from build123d import *

# Parameters (mm, degrees)
SKETCH1_R           = 10.16
BOSS_EXTRUDE4_DEPTH = 2.54
SKETCH1_7_R         = 10.16
BOSS_EXTRUDE5_DEPTH = 25.4
BOSS_EXTRUDE7_START = -27.94
SKETCH1_9_R         = 10.16
BOSS_EXTRUDE7_DEPTH = 2.54
FILLET1_R           = 0.508
FILLET2_R           = 0.508
FILLET3_R           = 0.508


with BuildPart() as part:
    # Sketch1 → Boss-Extrude4 (new body)
    # profile 1 of 4: a face of its own
    with BuildSketch(Plane(origin=(0, 0, 0), x_dir=(0, 0, -1), z_dir=(1, 0, 0))):
        with BuildLine():
            ThreePointArc((-12.743782522, 0.525454189), (-11.680659896, 5.122721879), (-9.018871744, 9.018871744))
            ThreePointArc((-9.018871744, 9.018871744), (-12.351999156, 6.704423948), (-16.283700751, 5.700367418))
            ThreePointArc((-16.283700751, 5.700367418), (-21.59, 0), (-16.283700751, -5.700367418))
            ThreePointArc((-16.283700751, -5.700367418), (-12.351999156, -6.704423948), (-9.018871744, -9.018871744))
            ThreePointArc((-9.018871744, -9.018871744), (-11.680659896, -5.122721879), (-12.743782522, -0.525454189))
            ThreePointArc((-12.743782522, -0.525454189), (-19.05, 0), (-12.743782522, 0.525454189))
        make_face()
    # profile 2 of 4: a face of its own
    with BuildSketch(Plane(origin=(0, 0, 0), x_dir=(0, 0, -1), z_dir=(1, 0, 0))):
        with BuildLine():
            ThreePointArc((12.743782522, -0.525454189), (12.7, 0), (12.743782522, 0.525454189))
            ThreePointArc((12.743782522, 0.525454189), (11.680659896, 5.122721879), (9.018871744, 9.018871744))
            ThreePointArc((9.018871744, 9.018871744), (6.704423948, 12.351999156), (5.700367418, 16.283700751))
            ThreePointArc((5.700367418, 16.283700751), (0, 21.59), (-5.700367418, 16.283700751))
            ThreePointArc((-5.700367418, 16.283700751), (-6.704423948, 12.351999156), (-9.018871744, 9.018871744))
            ThreePointArc((-9.018871744, 9.018871744), (-11.680659896, 5.122721879), (-12.743782522, 0.525454189))
            ThreePointArc((-12.743782522, 0.525454189), (-12.710964563, 0.263637542), (-12.7, 0))
            ThreePointArc((-12.7, 0), (-12.710964563, -0.263637542), (-12.743782522, -0.525454189))
            ThreePointArc((-12.743782522, -0.525454189), (-11.680659896, -5.122721879), (-9.018871744, -9.018871744))
            ThreePointArc((-9.018871744, -9.018871744), (-6.704423948, -12.351999156), (-5.700367418, -16.283700751))
            ThreePointArc((-5.700367418, -16.283700751), (0, -21.59), (5.700367418, -16.283700751))
            ThreePointArc((5.700367418, -16.283700751), (6.704423948, -12.351999156), (9.018871744, -9.018871744))
            ThreePointArc((9.018871744, -9.018871744), (11.680659896, -5.122721879), (12.743782522, -0.525454189))
        make_face()
        with BuildLine():
            ThreePointArc((0.525454189, -12.743782522), (2.423730807, -13.82410898), (3.175, -15.875))
            ThreePointArc((3.175, -15.875), (-2.05089102, -18.298730807), (-0.525454189, -12.743782522))
            ThreePointArc((-0.525454189, -12.743782522), (0, -12.7), (0.525454189, -12.743782522))
        make_face(mode=Mode.SUBTRACT)
        Circle(SKETCH1_R, mode=Mode.SUBTRACT)
        with BuildLine():
            ThreePointArc((-0.525454189, 12.743782522), (-2.05089102, 18.298730807), (3.175, 15.875))
            ThreePointArc((3.175, 15.875), (2.423730807, 13.82410898), (0.525454189, 12.743782522))
            ThreePointArc((0.525454189, 12.743782522), (0, 12.7), (-0.525454189, 12.743782522))
        make_face(mode=Mode.SUBTRACT)
    # profile 3 of 4: a face of its own
    with BuildSketch(Plane(origin=(0, 0, 0), x_dir=(0, 0, -1), z_dir=(1, 0, 0))):
        Circle(SKETCH1_R)
        Polygon((7.14375, -4.124445986), (7.14375, 4.124445986), (0, 8.248891971), (-7.14375, 4.124445986), (-7.14375, -4.124445986), (0, -8.248891971), align=None, mode=Mode.SUBTRACT)
    # profile 4 of 4: a face of its own
    with BuildSketch(Plane(origin=(0, 0, 0), x_dir=(0, 0, -1), z_dir=(1, 0, 0))):
        with BuildLine():
            ThreePointArc((12.743782522, 0.525454189), (16.138637542, 3.164035437), (19.05, 0))
            ThreePointArc((19.05, 0), (16.138637542, -3.164035437), (12.743782522, -0.525454189))
            ThreePointArc((12.743782522, -0.525454189), (11.680659896, -5.122721879), (9.018871744, -9.018871744))
            ThreePointArc((9.018871744, -9.018871744), (12.351999156, -6.704423948), (16.283700751, -5.700367418))
            ThreePointArc((16.283700751, -5.700367418), (21.59, 0), (16.283700751, 5.700367418))
            ThreePointArc((16.283700751, 5.700367418), (12.351999156, 6.704423948), (9.018871744, 9.018871744))
            ThreePointArc((9.018871744, 9.018871744), (11.680659896, 5.122721879), (12.743782522, 0.525454189))
        make_face()
    extrude(amount=BOSS_EXTRUDE4_DEPTH)

    # Sketch1<7> → Boss-Extrude5 (add)
    with BuildSketch(Plane(origin=(0, 0, 0), x_dir=(0, 0, -1), z_dir=(1, 0, 0))):
        Circle(SKETCH1_7_R)
        Polygon((7.14375, -4.124445986), (7.14375, 4.124445986), (0, 8.248891971), (-7.14375, 4.124445986), (-7.14375, -4.124445986), (0, -8.248891971), align=None, mode=Mode.SUBTRACT)
    extrude(amount=-BOSS_EXTRUDE5_DEPTH)

    # Sketch1<9> → Boss-Extrude7 (add)
    # profile 1 of 2: a face of its own
    with BuildSketch(Plane(origin=(0, 0, 0), x_dir=(0, 0, -1), z_dir=(1, 0, 0)).offset(BOSS_EXTRUDE7_START)):
        with BuildLine():
            ThreePointArc((12.743782522, -0.525454189), (12.7, 0), (12.743782522, 0.525454189))
            ThreePointArc((12.743782522, 0.525454189), (11.680659896, 5.122721879), (9.018871744, 9.018871744))
            ThreePointArc((9.018871744, 9.018871744), (6.704423948, 12.351999156), (5.700367418, 16.283700751))
            ThreePointArc((5.700367418, 16.283700751), (0, 21.59), (-5.700367418, 16.283700751))
            ThreePointArc((-5.700367418, 16.283700751), (-6.704423948, 12.351999156), (-9.018871744, 9.018871744))
            ThreePointArc((-9.018871744, 9.018871744), (-11.680659896, 5.122721879), (-12.743782522, 0.525454189))
            ThreePointArc((-12.743782522, 0.525454189), (-12.710964563, 0.263637542), (-12.7, 0))
            ThreePointArc((-12.7, 0), (-12.710964563, -0.263637542), (-12.743782522, -0.525454189))
            ThreePointArc((-12.743782522, -0.525454189), (-11.680659896, -5.122721879), (-9.018871744, -9.018871744))
            ThreePointArc((-9.018871744, -9.018871744), (-6.704423948, -12.351999156), (-5.700367418, -16.283700751))
            ThreePointArc((-5.700367418, -16.283700751), (0, -21.59), (5.700367418, -16.283700751))
            ThreePointArc((5.700367418, -16.283700751), (6.704423948, -12.351999156), (9.018871744, -9.018871744))
            ThreePointArc((9.018871744, -9.018871744), (11.680659896, -5.122721879), (12.743782522, -0.525454189))
        make_face()
        with BuildLine():
            ThreePointArc((0.525454189, -12.743782522), (2.423730807, -13.82410898), (3.175, -15.875))
            ThreePointArc((3.175, -15.875), (-2.05089102, -18.298730807), (-0.525454189, -12.743782522))
            ThreePointArc((-0.525454189, -12.743782522), (0, -12.7), (0.525454189, -12.743782522))
        make_face(mode=Mode.SUBTRACT)
        Circle(SKETCH1_9_R, mode=Mode.SUBTRACT)
        with BuildLine():
            ThreePointArc((-0.525454189, 12.743782522), (-2.05089102, 18.298730807), (3.175, 15.875))
            ThreePointArc((3.175, 15.875), (2.423730807, 13.82410898), (0.525454189, 12.743782522))
            ThreePointArc((0.525454189, 12.743782522), (0, 12.7), (-0.525454189, 12.743782522))
        make_face(mode=Mode.SUBTRACT)
    # profile 2 of 2: a face of its own
    with BuildSketch(Plane(origin=(0, 0, 0), x_dir=(0, 0, -1), z_dir=(1, 0, 0)).offset(BOSS_EXTRUDE7_START)):
        Circle(SKETCH1_9_R)
        Polygon((7.14375, -4.124445986), (7.14375, 4.124445986), (0, 8.248891971), (-7.14375, 4.124445986), (-7.14375, -4.124445986), (0, -8.248891971), align=None, mode=Mode.SUBTRACT)
    extrude(amount=BOSS_EXTRUDE7_DEPTH)

    # Fillet1
    fillet1_edges = [part.edges().sort_by_distance(p)[0] for p in [
        (2.54, 0, -21.59),
        (2.54, 9.018871744, -9.018871744),
        (2.54, 21.59, 0),
        (2.54, 9.018871744, 9.018871744),
        (2.54, 0, 21.59),
        (2.54, -9.018871744, 9.018871744),
        (2.54, -21.59, 0),
        (2.54, -9.018871744, -9.018871744),
    ]]
    fillet(fillet1_edges, radius=FILLET1_R)

    # Fillet2
    fillet2_edges = [part.edges().sort_by_distance(p)[0] for p in [
        (-26.67, -0.525454189, 12.743782522),
        (-26.67, 0.525454189, 12.743782522),
        (-26.67, 0.525454189, -12.743782522),
        (-26.67, -0.525454189, -12.743782522),
    ]]
    fillet(fillet2_edges, radius=FILLET2_R)

    # Fillet3
    fillet3_edges = [part.edges().sort_by_distance(p)[0] for p in [
        (-27.94, 0, 12.7),
        (-27.94, -5.146734512, 11.670099354),
        (-27.94, 5.146734512, -11.670099354),
        (-27.94, 0, -12.7),
        (-27.94, 0.527966167, -12.741322921),
        (-27.94, -0.527966167, -12.741322921),
        (-27.94, 0.527966167, 12.741322921),
        (-27.94, -0.527966167, 12.741322921),
        (-27.94, 5.146734512, 11.670099354),
        (-27.94, 21.59, 0),
        (-27.94, -5.146734512, -11.670099354),
        (-27.94, -21.59, 0),
        (-27.94, 12.351999156, 6.704423948),
        (-27.94, 12.351999156, -6.704423948),
        (-27.94, -12.351999156, -6.704423948),
        (-27.94, -12.351999156, 6.704423948),
    ]]
    fillet(fillet3_edges, radius=FILLET3_R - 0.0001)  # a hair under: the kernel refuses the full size


solid = part.part
CAD build for the part. Positions are in the model's coordinates, mm. A direction names the side the tool comes from. Coordinates: 2 decimals unless noted, no trailing zeros. Write each loop counter-clockwise with the first axis right and the second up, starting at its lowest first coordinate (ties: lowest second). Pieces come first, ordered by that corner, then holes. Notation, with made-up numbers: (70, 58.25) - (129, 58.25) arc R20 cw to (129, 76.25) - close; hole circle Ø8 at (22, 56.25). An arc over 180 degrees is marked (long way). Use a Markdown table: item, result. Add a question column.
Item 1: Band-saw the part on A-A, the plane x = -11. Give the cut face in (y, z), and give its area (3 significant figures).
Item 2: Drill centre lines: L1, parallel to X at y = 15, z = -5; L2, parallel to Z at x = -26, y = 0; L3, parallel to Y at x = -26, z = 5. Where is each one in solid material? Low to high. Write a range as from..to.
Item 3: Mould opens along X. For faces 1 (the face through (-26.43, 5.21, 11.64)), 2 (the face through (2.54, 6, 5)), 3 (the face through (-25.4, -8, -7)) say: pulls with the +X half, pulls with the -X half, needs draft (parallel to the pull), parting line crosses it, or undercut.
Item 4: 3-axis set-ups, long thin cutter, end or side, ignore diameter. For faces 4 (the face through (0, 10, 3)), 5 (the face through (-26.43, 5.086, -11.697)), 6 (the face through (-26.43, -5.21, -11.64)), 7 (the face through (-26.43, -5.086, 11.697)), 8 (the face through (-12.913, 6.216, 3.522)): which of +Z, -Z, +X, -X, +Y, -Y reach the whole face in a straight line?
Item 5: Flat gauge pins, fed straight in: pin 1 (5.5 mm diameter, centred on y = 15.875, z = 0, fed in from +X); pin 2 (9 mm diameter, centred on x = -10.5, y = -1, fed in from +Z); pin 3 (4 mm diameter, centred on x = -11, y = -1, fed in from -Z); pin 4 (8 mm diameter, centred on x = -11.5, y = 11, fed in from -Z). Where does each tip first touch, or does it go through?
Numbers:
| question | item | result |
|---|---|---|
| 1 | outline | circle Ø20.32 at (0, 0); hole (-8.25, 0) - (-4.12, -7.14) - (4.12, -7.14) - (8.25, 0) - (4.12, 7.14) - (-4.12, 7.14) - close |
| 1 | area | 148 mm2 |
| 2 | L1 | -27.94..-25.4, 0..2.54 |
| 2 | L2 | -12.7..-7.14, 7.14..12.7 |
| 2 | L3 | -18.64..-5.36, 5.36..18.64 |
| 3 | face 1 | needs draft |
| 3 | face 2 | pulls with the +X half |
| 3 | face 3 | undercut |
| 4 | face 4 | none |
| 4 | face 5 | -Z, -X, +Y |
| 4 | face 6 | -Z, -X, -Y |
| 4 | face 7 | +Z, -X, -Y |
| 4 | face 8 | +X, -X |
| 5 | pin 1 | through |
| 5 | pin 2 | z = 10.16 |
| 5 | pin 3 | z = -10.16 |
| 5 | pin 4 | z = -7.36 |
